Model file for the job. Use its own axes, mm. A direction names the side the tool comes from. Coordinates: 2 decimals unless noted, no trailing zeros. Order: outer loops, then holes, each group sorted by start corner. A loop starts at its lowest first (then second) coordinate and runs counter-clockwise, first axis right, second up. Notation, with made-up numbers: (-31.75, 5) -> (-27.75, 5) arc R22 ccw to (-27.75, 37) -> close; hole circle Ø1 at (43.25, 79). An arc over 180 degrees is marked (long way). Use CSV: the item, a comma, the result in double quotes. Start each with the question number.
(1) Probe L1, parallel to X at y = 2.85, z = 4.75; L2, parallel to X at y = 3.55, z = -1.25; L3, parallel to Z at x = 119.5, y = 1.65. List the from-to ranges inside material, lowest first.
(2) Cut at B-B on y = 3.8. Write the cut outline in (x, z), plus the area to 3 significant figures.
(3) Cut at C-C on z = 13. Write the cut outline in (x, y), plus the area to 3 significant figures.
(4) Pull direction X, two halves, no side cores. Call faces 3 (the cylindrical face through (134.92, 2.22, 5.86)), 4 (the flat face through (40.921, 2, 3)), 5 (the flat face through (-1, 2, -2.453)): pulls with the +X half, pulls with the -X half, needs draft (parallel to the pull), parting line crosses it, or undercut.
(5) Pin check, flat tips, straight feed: pin 1 Ø2 at (x, y) = (119.5, 1.5) entering from -Z; pin 2 Ø0.8 at (y, z) = (1.5, 10) entering from -X; pin 3 Ø2 at (y, z) = (3.5, 0.5) entering from +X. Stop position of each tip, or through.
(6) Tool access for faces 1 (the flat face through (-42.579, 2, 3)), 2 (the flat face through (41, 2, 14.547)): list every direction of +Z, -Z, +X, -X, +Y, -Y with a clear straight run to the whole face (end or side of a thin tool).
(7) Cut at A-A on z = 3. Write the cut outline in (x, y), plus the area to 3 significant figures.
```python
from build123d import *

# Parameters (mm, degrees)
BOSS_EXTRUDE1_DEPTH = 4.5


with BuildPart() as part:
    # Sketch1 → Boss-Extrude1 (new body)
    with BuildSketch(Plane(origin=(0, 0, 0), x_dir=(1, 0, 0), z_dir=(0, 1, 0))):
        with BuildLine():
            Line((40.921196651, 2.452604877), (83.421196651, 2.452604877))
            Line((83.421196651, 2.452604877), (87.921196651, 2.452604877))
            Line((87.921196651, 2.452604877), (117.921196651, 2.452604877))
            Line((117.921196651, 2.452604877), (117.921196651, -7.751372429))
            ThreePointArc((117.921196651, -7.751372429), (118.069207998, -7.899383776), (117.921196651, -8.047395123))
            Line((117.921196651, -8.047395123), (117.921196651, -10.547395123))
            Line((117.921196651, -10.547395123), (122.421196651, -10.547395123))
            Line((122.421196651, -10.547395123), (122.421196651, -8.047395123))
            ThreePointArc((122.421196651, -8.047395123), (122.268740731, -7.894939202), (122.421196651, -7.742483282))
            Line((122.421196651, -7.742483282), (122.421196651, 2.452604877))
            Line((122.421196651, 2.452604877), (126.421196651, 2.452604877))
            ThreePointArc((126.421196651, 2.452604877), (134.921196651, -6.047395123), (126.421196651, -14.547395123))
            Line((126.421196651, -14.547395123), (-46.578803349, -14.547395123))
            ThreePointArc((-46.578803349, -14.547395123), (-55.078803349, -6.047395123), (-46.578803349, 2.452604877))
            Line((-46.578803349, 2.452604877), (-42.578803349, 2.452604877))
            Line((-42.578803349, 2.452604877), (-42.578803349, -7.749399248))
            ThreePointArc((-42.578803349, -7.749399248), (-42.429805412, -7.898397185), (-42.578803349, -8.047395123))
            Line((-42.578803349, -8.047395123), (-42.578803349, -10.547395123))
            Line((-42.578803349, -10.547395123), (-38.078803349, -10.547395123))
            Line((-38.078803349, -10.547395123), (-38.078803349, -8.047395123))
            ThreePointArc((-38.078803349, -8.047395123), (-38.227801286, -7.898397185), (-38.078803349, -7.749399248))
            Line((-38.078803349, -7.749399248), (-38.078803349, 2.452604877))
            Line((-38.078803349, 2.452604877), (-8.078803349, 2.452604877))
            Line((-8.078803349, 2.452604877), (-3.578803349, 2.452604877))
            Line((-3.578803349, 2.452604877), (36.421196651, 2.452604877))
            Line((36.421196651, 2.452604877), (36.421196651, -7.747669694))
            ThreePointArc((36.421196651, -7.747669694), (36.571059365, -7.897532409), (36.421196651, -8.047395123))
            Line((36.421196651, -8.047395123), (36.421196651, -10.547395123))
            Line((36.421196651, -10.547395123), (40.921196651, -10.547395123))
            Line((40.921196651, -10.547395123), (40.921196651, -8.047395123))
            ThreePointArc((40.921196651, -8.047395123), (40.771333937, -7.897532409), (40.921196651, -7.747669694))
            Line((40.921196651, -7.747669694), (40.921196651, 2.452604877))
        make_face()
    extrude(amount=BOSS_EXTRUDE1_DEPTH)


solid = part.part
```
Outcome:
1,L1,"-54.98 to -42.58, -38.08 to 36.42, 40.92 to 117.92, 122.42 to 134.82"
1,L2,"-50.94 to -42.58, -38.08 to 36.42, 40.92 to 117.92, 122.42 to 130.78"
1,L3,"10.55 to 14.55"
2,outline,"(-46.58, -2.45) -> (-42.58, -2.45) -> (-42.58, 7.75) arc R0.15 ccw to (-42.58, 8.05) -> (-42.58, 10.55) -> (-38.08, 10.55) -> (-38.08, 8.05) arc R0.15 ccw to (-38.08, 7.75) -> (-38.08, -2.45) -> (36.42, -2.45) -> (36.42, 7.75) arc R0.15 ccw to (36.42, 8.05) -> (36.42, 10.55) -> (40.92, 10.55) -> (40.92, 8.05) arc R0.15 ccw to (40.92, 7.75) -> (40.92, -2.45) -> (117.92, -2.45) -> (117.92, 7.75) arc R0.15 ccw to (117.92, 8.05) -> (117.92, 10.55) -> (122.42, 10.55) -> (122.42, 8.05) arc R0.15 ccw to (122.42, 7.74) -> (122.42, -2.45) -> (126.42, -2.45) arc R8.5 ccw to (126.42, 14.55) -> (-46.58, 14.55) arc R8.5 ccw to start"
2,area,"2,990 mm2"
3,outline,"(-51.47, 0) -> (131.31, 0) -> (131.31, 4.5) -> (-51.47, 4.5) -> close"
3,area,"823 mm2"
4,face 3,"pulls with the +X half"
4,face 4,"undercut"
4,face 5,"needs draft"
5,pin 1,"z = 10.55"
5,pin 2,"x = -54.3"
5,pin 3,"x = 133.6"
6,face 1,"-Z, +Y, -Y"
6,face 2,"+Z, +X, -X, +Y, -Y"
7,outline,"(-54.51, 0) -> (-42.58, 0) -> (-42.58, 4.5) -> (-54.51, 4.5) -> close; (-38.08, 0) -> (36.42, 0) -> (36.42, 4.5) -> (-38.08, 4.5) -> close; (40.92, 0) -> (117.92, 0) -> (117.92, 4.5) -> (40.92, 4.5) -> close; (122.42, 0) -> (134.36, 0) -> (134.36, 4.5) -> (122.42, 4.5) -> close"
7,area,"789 mm2"
